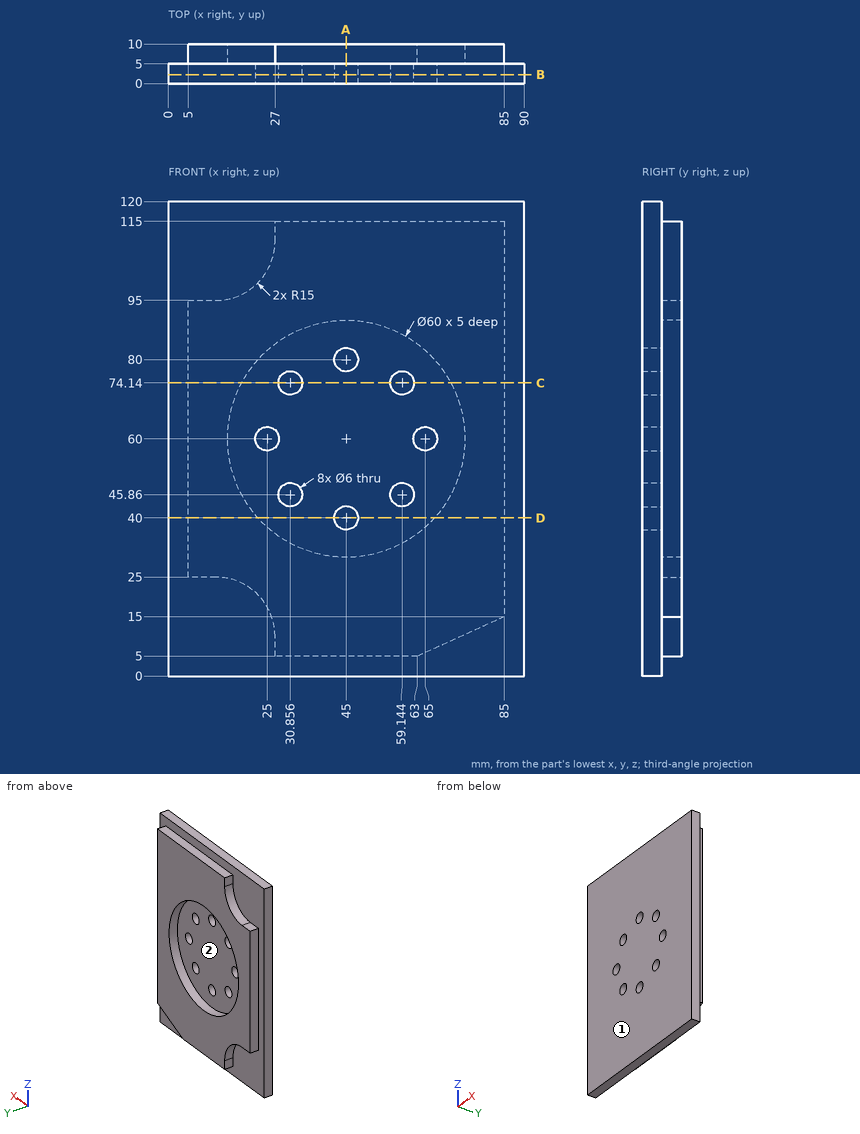
Drawing for the job (mm, zero at the part's lowest x, y, z). Give positions to 0.01 mm unless a question says otherwise; leave off trailing zeros. Loops run counter-clockwise (first coordinate to the right, second up) from the corner with the lowest first, then second, coordinate; pieces in that order, holes last. Notation, with made-up numbers: M -20,-14 L 4,-14 A21 ccw 4,25 Z; hole C -32.75,-2 d10. An arc over 180 degrees is marked long. Use one line per item in the form item = value.
Item 1: Slice it at B-B (y = 2.25). Count the separate pieces of the cut face and the enclosed holes in it, plus the area to 3 significant figures.
Determined:
separate_pieces = 1
enclosed_holes = 8
area = 10,600 mm2
Item 2: Slice it at C-C (z = 74.14). List the corners of the cut face in (x, y).
Determined:
outline = M 0,0 L 27.86,0 L 27.86,5 L 18.54,5 L 18.54,10 L 5,10 L 5,5 L 0,5 Z; M 33.86,0 L 56.14,0 L 56.14,5 L 33.86,5 Z; M 62.14,0 L 90,0 L 90,5 L 85,5 L 85,10 L 71.46,10 L 71.46,5 L 62.14,5 Z
Item 3: Drill centre lines: probe 1 along Z at (x, y) = (45, 3.1); probe 2 along Z at (x, y) = (45, 7.45); probe 3 along Z at (x, y) = (67.5, 9.75) (1 decimal). Where is each one in solid material? Low to high. Write a range as from..to.
Determined:
probe_1 = 0..37, 43..77, 83..120
probe_2 = 5..30, 90..115
probe_3 = 7..40.2, 79.8..115
Item 4: Flat gauge pins, fed straight in: pin 1 (4 mm diameter, centred on x = 55.5, y = 8, fed in from +Z); pin 2 (18 mm diameter, centred on x = 38.5, z = 54, fed in from +Y); pin 3 (1.5 mm diameter, centred on y = 7.5, z = 112.5, fed in from -X). Where does each tip first touch, or does it go through?
Determined:
pin_1 = 115
pin_2 = 5
pin_3 = 27
Item 5: Two-plate mould, pull along X, no slides. Class the marked faces 1 and 2: pulls with the +X half, pulls with the -X half, needs draft (parallel to the pull), parting line crosses it, or undercut.
Determined:
face_1 = needs draft
face_2 = undercut
Item 6: Slice it at D-D (z = 40). List the corners of the cut face in (x, y).
Determined:
outline = M 0,0 L 42,0 L 42,5 L 22.64,5 L 22.64,10 L 5,10 L 5,5 L 0,5 Z; M 48,0 L 90,0 L 90,5 L 85,5 L 85,10 L 67.36,10 L 67.36,5 L 48,5 Z
Item 7: Slice it at A-A (x = 45). List the corners of the cut face in (y, z).
Determined:
outline = M 0,0 L 5,0 L 5,5 L 10,5 L 10,30 L 5,30 L 5,37 L 0,37 Z; M 0,43 L 5,43 L 5,77 L 0,77 Z; M 0,83 L 5,83 L 5,90 L 10,90 L 10,115 L 5,115 L 5,120 L 0,120 Z
